Source: CAD feature listing. Evaluate the final solid. Frame: model axes, mm. A direction names the side the tool comes from. Give positions to 0.01 mm unless a question says otherwise; leave off trailing zeros. Order: outer loops, then holes, each group sorted by start corner. A loop starts at its lowest first (then second) coordinate and runs counter-clockwise, first axis right, second up. Notation, with made-up numbers: M 51.25,49 L 82.25,49 A21 ccw 82.25,60 Z; hole C 69,4.5 d8. An arc over 180 degrees is marked long. Answer in a Markdown table with one row per item. Add a question column.
(1) Pin query (flat end, axial travel): P1, Ø1.5, axis at x = 0.5, z = 7, coming from the -Y side; P2, Ø6, axis at y = -6, z = -6, coming from the -X side; P3, Ø1.2, axis at x = 1.5, y = 16, coming from the +Z side; P4, Ø0.8, axis at x = 1.5, z = 8.5, coming from the +Y side. Return the tip coordinate at first contact, or that it passes through.
(2) Section query A-A, the plane x = 1.65. Return loops of the section in (y, z).
(3) Section query B-B, the plane z = 11.25. Return loops of the section in (x, y).
(4) Material intervals for line 1 along Y through (x, z) = (1.2, -7.5); line 2 along Z through (x, y) = (1.5, 15.5), sorted ascending.
(5) Set-up query: faces 1 (the face through (0, 0, 3)), 2 (the face through (1, 16, -2.5)), 3 (the face through (1, -15, -6)), 4 (the face through (1, 15, 9)), 5 (the face through (1, -15, 10)). Return all of +Z, -Z, +X, -X, +Y, -Y with unobstructed straight access to the full face (end or side cutting, diameter ignored); none if empty.
from build123d import *

# Parameters (mm, degrees)
SKETCH1_5_W         = 3.85
SKETCH1_5_H         = 30
SKETCH1_5_W_2       = 6.42
BOSS_EXTRUDE4_DEPTH = 2.5


with BuildPart() as part:
    # Sketch1_5 → Boss-Extrude4 (new body)
    with BuildSketch(Plane(origin=(0, 0, 0), x_dir=(0, 0, -1), z_dir=(1, 0, 0))):
        with Locations((-8.105, 0)):
            Rectangle(SKETCH1_5_W, SKETCH1_5_H)
        Polygon((-6.18, 15), (-6.18, -15), (-2.5, -15), (-2.5, -17.5), (2.5, -17.5), (2.5, -15), (10.03, -15), (10.03, 15), (2.5, 15), (2.5, 17.5), (-2.5, 17.5), (-2.5, 15), align=None)
        with Locations((-13.24, 0)):
            Rectangle(SKETCH1_5_W_2, SKETCH1_5_H)
    extrude(amount=BOSS_EXTRUDE4_DEPTH)


solid = part.part
Values follow:
| question | item | result |
|---|---|---|
| 1 | P1 | stops at y = -15 |
| 1 | P2 | stops at x = 0 |
| 1 | P3 | stops at z = 2.5 |
| 1 | P4 | stops at y = 15 |
| 2 | outline | M -17.5,-2.5 L -15,-2.5 L -15,-10.03 L 15,-10.03 L 15,-2.5 L 17.5,-2.5 L 17.5,2.5 L 15,2.5 L 15,16.45 L -15,16.45 L -15,2.5 L -17.5,2.5 Z |
| 3 | outline | M 0,-15 L 2.5,-15 L 2.5,15 L 0,15 Z |
| 4 | line 1 | y = -15 to 15 |
| 4 | line 2 | z = -2.5 to 2.5 |
| 5 | face 1 | +Z, -Z, -X, +Y, -Y |
| 5 | face 2 | -Z, +X, -X, +Y |
| 5 | face 3 | -Z, +X, -X, -Y |
| 5 | face 4 | +Z, +X, -X, +Y |
| 5 | face 5 | +Z, +X, -X, -Y |
